Part model, mm, in its own coordinate system. Face numbers are marked on the shaded views. A direction names the side the tool comes from. Round coordinates to 2 decimals unless told otherwise and drop trailing zeros. Loops run counter-clockwise (first coordinate to the right, second up) from the corner with the lowest first, then second, coordinate; pieces in that order, holes last.
1) Drop flat-ended pins along their axis: P1, Ø2, axis at x = 64.5, y = 55.5, coming from the -Z side; P2, Ø2, axis at x = 89.5, y = 17, coming from the +Z side; P3, Ø1, axis at y = 1, z = 14, coming from the +X side; P4, Ø1, axis at x = 68.5, y = 10.5, coming from the +Z side. Give the stop position or say it passes through.
2) Probe line 1 (Y direction, x = 6.5, z = 1.15); line 2 (Y direction, x = 6.5, z = 5.75); line 3 (Y direction, x = 83, z = 11.25). List the from-to ranges inside material, lowest first.
3) Band-saw the part on B-B, the plane z = 5.75. State how many separate pieces and enclosed holes the cut face has, then the cut area to 3 significant figures.
4) 3-axis set-ups, long thin cutter, end or side, ignore diameter. For the marked faces 4 and 5: which of +Z, -Z, +X, -X, +Y, -Y reach the whole face in a straight line?
5) Band-saw the part on D-D, the plane x = 28. Write the cut outline in (y, z).
6) Mould opens along Y. For the marked faces 1, 2 and 3 say: +Y half, -Y half, draft (parallel to the pull), parting line (faces both ways), or undercut.
7) Band-saw the part on C-C, the plane x = 64.5. Write the cut outline in (y, z).
8) Band-saw the part on A-A, the plane y = 55.5. Write the cut outline in (x, z).
from build123d import *

# Parameters (mm, degrees)
F0_W           = 91
F0_H           = 62
F0_W_2         = 87
F0_H_2         = 58
F1_DEPTH       = 2
F2_DEPTH       = 19
F3_R           = 2.75
F3_R_2         = 1.25
F4_DEPTH       = 5
F5_DEPTH       = 2.001
F6_W           = 3
F6_H           = 15.1
F6_H_2         = 15.9
F6_W_2         = 9
F6_H_3         = 2
F6_W_3         = 17
F6_W_4         = 8
F7_DEPTH       = 12
F8_R           = 2
F9_W           = 2
F9_H           = 15.6
F10_DEPTH      = 3
F10_DEPTH_BACK = 1


# Not quite as in the source:
# - a feature names something its author has since deleted; it is built from what else it names


with BuildPart() as f1:
    # F0 (on Top) → F1 (new body)
    with BuildSketch(Plane.XY):
        with Locations((45.5, 31)):
            Rectangle(F0_W, F0_H)
        with Locations((45.5, 31)):
            Rectangle(F0_W_2, F0_H_2, mode=Mode.SUBTRACT)
        with Locations((45.5, 31)):
            Rectangle(F0_W_2, F0_H_2)
    extrude(amount=F1_DEPTH)

    # F0 (on Top) → F2 (join)
    with BuildSketch(Plane.XY):
        with Locations((45.5, 31)):
            Rectangle(F0_W, F0_H)
        with Locations((45.5, 31)):
            Rectangle(F0_W_2, F0_H_2, mode=Mode.SUBTRACT)
    extrude(amount=F2_DEPTH)

    # F3 (on face) → F4 (join)
    with BuildSketch(Plane.XY.offset(2)):
        with Locations((6.5, 55.5)):
            Circle(F3_R)
        with Locations((6.5, 55.5)):
            Circle(F3_R_2, mode=Mode.SUBTRACT)
        with Locations((64.5, 55.5)):
            Circle(F3_R)
        with Locations((64.5, 55.5)):
            Circle(F3_R_2, mode=Mode.SUBTRACT)
        with Locations((64.5, 6.5)):
            Circle(F3_R)
        with Locations((64.5, 6.5)):
            Circle(F3_R_2, mode=Mode.SUBTRACT)
        with Locations((6.5, 6.5)):
            Circle(F3_R)
        with Locations((6.5, 6.5)):
            Circle(F3_R_2, mode=Mode.SUBTRACT)
    extrude(amount=F4_DEPTH)

    # F5 (cut, through all): faces of the model
    f5_faces = [f1.faces().sort_by_distance(p)[0] for p in [
        (6.5, 55.5, 2),
        (64.5, 55.5, 2),
        (64.5, 6.5, 2),
        (6.5, 6.5, 2),
    ]]
    extrude(f5_faces, amount=-F5_DEPTH, mode=Mode.SUBTRACT)

    # F6 (on face) → F7 (cut, through all)
    with BuildSketch(Plane.XY.offset(19)):
        with Locations((89.5, 49.95)):
            Rectangle(F6_W, F6_H)
        with Locations((89.5, 30.95)):
            Rectangle(F6_W, F6_H)
        with Locations((89.5, 13.25)):
            Rectangle(F6_W, F6_H_2)
        with Locations((13.55, 1)):
            Rectangle(F6_W_2, F6_H_3)
        with Locations((35, 1)):
            Rectangle(F6_W_3, F6_H_3)
        with Locations((57.25, 1)):
            Rectangle(F6_W_4, F6_H_3)
    extrude(amount=-F7_DEPTH, mode=Mode.SUBTRACT)

    # F8
    f8_edges = [f1.edges().sort_by_distance(p)[0] for p in [
        (91, 0, 9.5),
        (91, 62, 9.5),
        (0, 0, 9.5),
        (0, 62, 9.5),
    ]]
    fillet(f8_edges, radius=F8_R)

    # F9 (on face) → F10 (cut, two sides)
    with BuildSketch(Plane.XY.offset(7)) as f10_sk:
        with Locations((1, 31.7)):
            Rectangle(F9_W, F9_H)
    extrude(amount=-F10_DEPTH, mode=Mode.SUBTRACT)
    extrude(f10_sk.sketch, amount=F10_DEPTH_BACK, mode=Mode.SUBTRACT)


solid = f1.part
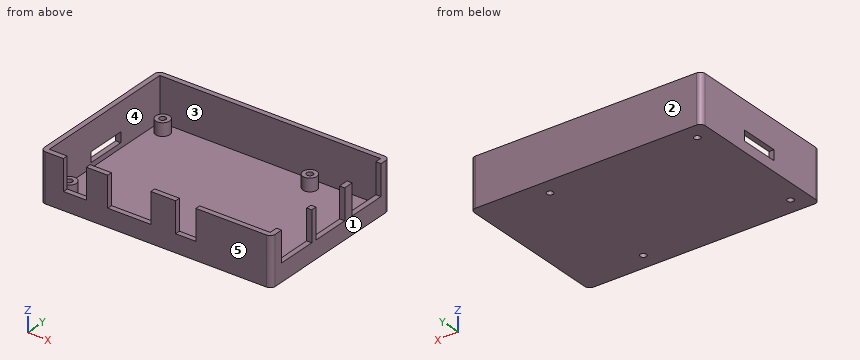
Reported:
1. P1: passes through
1. P2: stops at z = 7
1. P3: stops at x = 90.94
1. P4: stops at z = 2
2. line 1: y = 0 to 5.25, 7.75 to 54.25, 56.75 to 62
2. line 2: y = 0 to 2, 3.75 to 5.25, 7.75 to 9.25, 52.75 to 54.25, 56.75 to 58.25, 60 to 62
2. line 3: y = 0 to 2, 60 to 62
3. separate pieces: 5
3. enclosed holes: 4
3. area: 637 mm2
4. face 4: +Z
4. face 5: +Z, -Z, +X, -X, -Y
5. outline: (0, 0) - (62, 0) - (62, 19) - (60, 19) - (60, 2) - (2, 2) - (2, 7) - (0, 7) - close
6. face 1: draft
6. face 2: +Y half
6. face 3: undercut
7. outline: (0, 0) - (5.25, 0) - (5.25, 7) - (3.75, 7) - (3.75, 2) - (2, 2) - (2, 19) - (0, 19) - close; (7.75, 0) - (54.25, 0) - (54.25, 7) - (52.75, 7) - (52.75, 2) - (9.25, 2) - (9.25, 7) - (7.75, 7) - close; (56.75, 0) - (62, 0) - (62, 19) - (60, 19) - (60, 2) - (58.25, 2) - (58.25, 7) - (56.75, 7) - close
8. outline: (0, 0) - (5.25, 0) - (5.25, 7) - (3.75, 7) - (3.75, 2) - (2, 2) - (2, 19) - (0, 19) - close; (7.75, 0) - (63.25, 0) - (63.25, 7) - (61.75, 7) - (61.75, 2) - (9.25, 2) - (9.25, 7) - (7.75, 7) - close; (65.75, 0) - (91, 0) - (91, 7) - (89, 7) - (89, 2) - (67.25, 2) - (67.25, 7) - (65.75, 7) - close
